The model under review builds one solid part; all positions refer to its coordinate system, in mm. Face numbers are marked on the shaded views. A direction names the side the tool comes from. Round coordinates to 2 decimals unless told otherwise and drop trailing zeros. Write each loop counter-clockwise with the first axis right and the second up, starting at its lowest first coordinate (ties: lowest second). Pieces come first, ordered by that corner, then holes. Notation, with made-up numbers: (9, -39) -> (63, -39) arc R10 cw to (63, -30) -> close; hole circle Ø10 at (-26, 82.25). An arc over 180 degrees is marked (long way). Return JSON: item names as keys, results as strings. Group by question number.
1. Clearance check with flat-ended pins moving along their axes: P1, Ø1.2, axis at x = 5.5, z = 26, coming from the +Y side; P2, Ø5, axis at x = 2, z = 61.5, coming from the +Y side. State where each tip first meets the part, or that it passes through.
2. Take a section at B-B, the plane y = 28.5. Write out the cut boundary in (x, z), then the cut area to 3 significant figures.
3. Mouldability with a two-part tool opening along Z and no side actions: class the marked faces 3, 4 and 5 as pulls with the +Z half, pulls with the -Z half, needs draft (parallel to the pull), parting line crosses it, or undercut.
4. Take a section at A-A, the plane z = 68.5. Write out the cut boundary in (x, y), then the cut area to 3 significant figures.
5. Take a section at D-D, the plane x = 15. Write out the cut boundary in (y, z), then the cut area to 3 significant figures.
6. For line 1 along X through (y, z) = (24.5, 21); line 2 along Z through (x, y) = (14, 14.5); line 3 along Z through (x, y) = (0, 8.5), list the stretches that pass through material, from the lowest coordinate up. Write a range as from..to.
7. Take a section at C-C, the plane z = 6. Write out the cut boundary in (x, y).
8. Tool access review of the marked faces 1 and 2: name each direction out of +Z, -Z, +X, -X, +Y, -Y from which nothing blocks a thin tool from reaching the whole face with its end or side.
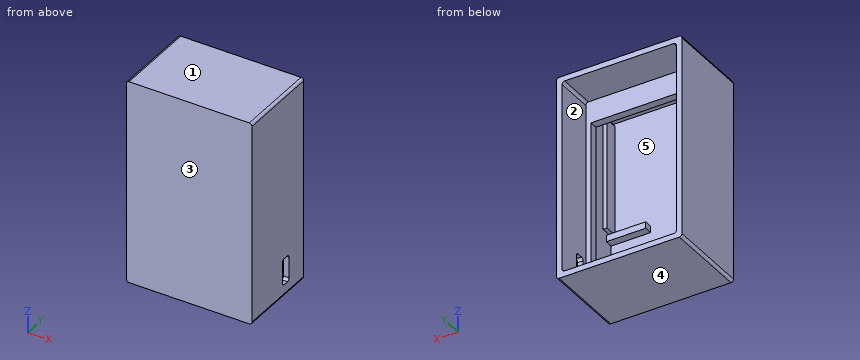
from build123d import *

# Parameters (mm, degrees)
PCB_DIMENSIONS_W    = 47.716732244
PCB_DIMENSIONS_H    = 77.636732244
BOSS_EXTRUDE3_DEPTH = 1.5
SKETCH5_W           = 47.716732244
SKETCH5_H           = 77.636732244
SKETCH5_W_2         = 43.474091557
SKETCH5_H_2         = 73.394091557
BOSS_EXTRUDE5_DEPTH = 30
FILLET1_R           = 1
SKETCH9_W           = 1.93805105
SKETCH9_H           = 42
SKETCH9_W_2         = 1.938051049
BOSS_EXTRUDE6_DEPTH = 5
SKETCH14_W          = 15
SKETCH14_H          = 2.5
BOSS_EXTRUDE7_DEPTH = 3
SKETCH15_W          = 75.636732244
SKETCH15_H          = 3
BOSS_EXTRUDE8_DEPTH = 46
SKETCH17_W          = 39.522771214
SKETCH17_H          = 62.982276128
CUT_EXTRUDE1_DEPTH  = 3
CUT_EXTRUDE2_DEPTH  = 3
SKETCH19_W          = 10
SKETCH19_H          = 4
CUT_EXTRUDE3_DEPTH  = 10
FILLET2_R           = 1
SCALE1_SCALE        = 0.99


with BuildPart() as part:
    # PCB Dimensions → Boss-Extrude3 (new body)
    with BuildSketch(Plane(origin=(0, 0, 0), x_dir=(1, 0, 0), z_dir=(0, 1, 0))):
        with Locations((20.322832216, -35.282832216)):
            Rectangle(PCB_DIMENSIONS_W, PCB_DIMENSIONS_H)
    extrude(amount=BOSS_EXTRUDE3_DEPTH)

    # Sketch5 → Boss-Extrude5 (add)
    with BuildSketch(Plane(origin=(0, 1.5, 0), x_dir=(1, 0, 0), z_dir=(0, 1, 0))):
        with Locations((20.322832216, -35.282832216)):
            Rectangle(SKETCH5_W, SKETCH5_H)
        with Locations((20.322832217, -35.282832217)):
            Rectangle(SKETCH5_W_2, SKETCH5_H_2, mode=Mode.SUBTRACT)
    extrude(amount=BOSS_EXTRUDE5_DEPTH)

    # Fillet1
    fillet1_edges = [part.edges().sort_by_distance(p)[0] for p in [
        (42.059877995, 16.5, -1.414213562),
        (-1.414213562, 16.5, -1.414213562),
        (-1.414213562, 16.5, 71.979877995),
        (42.059877995, 16.5, 71.979877995),
        (44.181198338, 15.75, 74.101198338),
        (-3.535533906, 15.75, 74.101198338),
        (-3.535533906, 15.75, -3.535533906),
        (44.181198338, 15.75, -3.535533906),
    ]]
    fillet(fillet1_edges, radius=FILLET1_R)

    # Sketch9 → Boss-Extrude6 (add)
    with BuildSketch(Plane(origin=(0, 1.5, 0), x_dir=(1, 0, 0), z_dir=(0, 1, 0))):
        with Locations((-0.88911969, -49.979881394)):
            Rectangle(SKETCH9_W, SKETCH9_H)
        with Locations((41.534784122, -49.979881394)):
            Rectangle(SKETCH9_W_2, SKETCH9_H)
    extrude(amount=BOSS_EXTRUDE6_DEPTH)

    # Sketch14 → Boss-Extrude7 (add)
    with BuildSketch(Plane(origin=(0, 1.5, 0), x_dir=(1, 0, 0), z_dir=(0, 1, 0))):
        with Locations((6.085786438, -26.529881394)):
            Rectangle(SKETCH14_W, SKETCH14_H)
        with Locations((34.559877995, -26.529881394)):
            Rectangle(SKETCH14_W, SKETCH14_H)
    extrude(amount=BOSS_EXTRUDE7_DEPTH)

    # Sketch15 → Boss-Extrude8 (add)
    with BuildSketch(Plane(origin=(44.181198338, 0, 0), x_dir=(0, 0, -1), z_dir=(1, 0, 0))):
        with Locations((-35.282832216, 15.5)):
            Rectangle(SKETCH15_W, SKETCH15_H)
    extrude(amount=-BOSS_EXTRUDE8_DEPTH)

    # Sketch17 → Cut-Extrude1 (cut)
    with BuildSketch(Plane(origin=(0, 17, 0), x_dir=(1, 0, 0), z_dir=(0, 1, 0))):
        with Locations((20.322832216, -32.052584673)):
            Rectangle(SKETCH17_W, SKETCH17_H)
    extrude(amount=-CUT_EXTRUDE1_DEPTH, mode=Mode.SUBTRACT)

    # Sketch18 → Cut-Extrude2 (cut)
    with BuildSketch(Plane(origin=(0, 17, 0), x_dir=(1, 0, 0), z_dir=(0, 1, 0))):
        with BuildLine():
            Line((-1.414213562, -9.585786438), (28.585786438, -9.585786438))
            Line((28.585786438, -9.585786438), (28.585786438, 1.414213562))
            Line((28.585786438, 1.414213562), (-0.414213562, 1.414213562))
            ThreePointArc((-0.414213562, 1.414213562), (-1.121320344, 1.121320344), (-1.414213562, 0.414213562))
            Line((-1.414213562, 0.414213562), (-1.414213562, -9.585786438))
        make_face()
    extrude(amount=-CUT_EXTRUDE2_DEPTH, mode=Mode.SUBTRACT)

    # Sketch19 → Cut-Extrude3 (cut)
    with BuildSketch(Plane(origin=(44.181198338, 0, 0), x_dir=(0, 0, -1), z_dir=(1, 0, 0))):
        with Locations((-5.964466094, 20.65)):
            Rectangle(SKETCH19_W, SKETCH19_H)
    extrude(amount=-CUT_EXTRUDE3_DEPTH, mode=Mode.SUBTRACT)

    # Fillet2
    fillet2_edges = [part.edges().sort_by_distance(p)[0] for p in [
        (43.120538167, 22.65, 0.964466094),
        (43.120538167, 18.65, 0.964466094),
        (43.120538167, 18.65, 10.964466094),
        (43.120538167, 22.65, 10.964466094),
    ]]
    fillet(fillet2_edges, radius=FILLET2_R)


with BuildPart() as part_1:
    # Scale1: scaled about (20.339813051, 12.239416384, 37.051144502)
    add(part.part.scale(SCALE1_SCALE).moved(Location((0.203398131, 0.122394164, 0.370511445))))


solid = part_1.part
Output:
{
 "1": {"P1": "stops at y = 4.58", "P2": "stops at y = 16.95"},
 "2": {"outline": "(-3.3, -2.14) arc R0.99 ccw to (-2.31, -3.13) -> (42.95, -3.13) arc R0.99 ccw to (43.94, -2.14) -> (43.94, 72.74) arc R0.99 ccw to (42.95, 73.73) -> (-2.31, 73.73) arc R0.99 ccw to (-3.3, 72.74) -> close; hole (-1.2, -0.04) arc R0.99 ccw to (-0.21, -1.03) -> (40.85, -1.03) arc R0.99 ccw to (41.84, -0.04) -> (41.84, 70.64) arc R0.99 ccw to (40.85, 71.63) -> (-0.21, 71.63) arc R0.99 ccw to (-1.2, 70.64) -> close", "area": "504 mm^2"},
 "3": {"face 3": "needs draft", "face 4": "pulls with the -Z half", "face 5": "undercut"},
 "4": {"outline": "(-3.3, 0.12) -> (43.94, 0.12) -> (43.94, 31.31) -> (41.84, 31.31) -> (41.84, 16.95) -> (-1.2, 16.95) -> (-1.2, 31.31) -> (-3.3, 31.31) -> close; hole (-1.2, 6.56) -> (0.28, 6.56) -> (0.28, 1.61) -> (40.36, 1.61) -> (40.36, 6.56) -> (41.84, 6.56) -> (41.84, 13.98) -> (-1.2, 13.98) -> close", "area": "337 mm^2"},
 "5": {"outline": "(0.12, -3.13) -> (31.31, -3.13) -> (31.31, -1.03) -> (1.61, -1.03) -> (1.61, 71.63) -> (13.98, 71.63) -> (13.98, 63.28) -> (16.95, 63.28) -> (16.95, 71.63) -> (31.31, 71.63) -> (31.31, 73.73) -> (0.12, 73.73) -> close", "area": "264 mm^2"},
 "6": {"line 1": "x = -3.3..-1.2, 41.84..43.94", "line 2": "z = -3.13..-1.03, 63.28..73.73", "line 3": "z = -3.13..-1.03, 71.63..73.73"},
 "7": {"outline": "(-3.3, 0.12) -> (43.94, 0.12) -> (43.94, 18.59) -> (41.84, 18.59) -> (41.84, 16.95) -> (39.89, 16.95) -> (39.89, 13.98) -> (41.84, 13.98) -> (41.84, 1.61) -> (-1.2, 1.61) -> (-1.2, 31.31) -> (-3.3, 31.31) -> close; (41.84, 22.55) -> (43.94, 22.55) -> (43.94, 31.31) -> (41.84, 31.31) -> close"},
 "8": {"face 1": "+Z, +X, -X, +Y, -Y", "face 2": "+Y"}
}
